Design review of the part built by this model. Coordinates are the model's own, in mm. A direction names the side the tool comes from. Coordinates: 2 decimals unless noted, no trailing zeros. Loops run counter-clockwise (first coordinate to the right, second up) from the corner with the lowest first, then second, coordinate; pieces in that order, holes last. Notation, with made-up numbers: (37, -32) -> (68, -32) arc R19 ccw to (68, -27) -> close; hole circle Ø2 at (2, 23). An arc over 180 degrees is marked (long way). Use a Markdown table: item, result. Add a question column.
Q1. Take a section at C-C on y = -12. Write out the cut boundary in (x, z) (3 decimals).
Q2. Take a section at D-D on z = 4.75. Write out the cut boundary in (x, y).
Q3. For probe 1 along Y at (x, z) = (19.5, -6); probe 2 along Z at (x, y) = (-4, -34); probe 3 along X at (y, z) = (-42, -5.25), list the stretches that pass through material, from the lowest coordinate up.
Q4. For faces 1 (the face through (11, -48, 9.525)), 2 (the face through (-9.516, -25.044, 0.419)), 3 (the face through (12, -50.8, 0)), list the 3-axis set-ups (+Z, -Z, +X, -X, +Y, -Y) from which the entire face can be reached by the end or side of a thin tool; tool diameter is ignored.
Q5. Take a section at B-B on x = 5. Write out the cut boundary in (y, z) (3 decimals), plus the area to 3 significant figures.
Q6. Clearance check with flat-ended pins moving along their axes: pin 1 Ø1.5 at (x, y) = (1.5, -31) entering from +Z; pin 2 Ø5 at (x, y) = (3, -41.5) entering from -Z; pin 3 Ø9.5 at (x, z) = (19.5, 4) entering from +Y. State where each tip first meets the part, or that it passes through.
Q7. Take a section at A-A on z = 0. Write out the cut boundary in (x, y) (3 decimals).
from build123d import *

# Parameters (mm, degrees)
F0_R     = 9.525
F1_DEPTH = 50.8
F3_DEPTH = 6.35
F4_W     = 3.175
F4_H     = 6.35
F5_DEPTH = 0.381


with BuildPart() as f1:
    # F0 (on Front) → F1 (new body)
    with BuildSketch(Plane.XZ):
        Circle(F0_R)
    extrude(amount=F1_DEPTH)

    # F2 (on face) → F3 (join)
    with BuildSketch(Plane.XZ.offset(50.8)):
        with BuildLine():
            Line((0, -9.525), (25.4, -9.525))
            ThreePointArc((25.4, -9.525), (34.925, 0), (25.4, 9.525))
            Line((25.4, 9.525), (0, 9.525))
            ThreePointArc((0, 9.525), (9.525, 0), (0, -9.525))
        make_face()
    extrude(amount=-F3_DEPTH)

    # F4 (on face) → F5 (join)
    with BuildSketch(Plane.XY.offset(9.525)):
        with Locations((23.8125, -47.625)):
            Rectangle(F4_W, F4_H)
    extrude(amount=F5_DEPTH)


solid = f1.part
Answer list:
| question | item | result |
|---|---|---|
| 1 | outline | circle Ø19.05 at (0, 0) |
| 2 | outline | (-8.26, -50.8) -> (33.66, -50.8) -> (33.66, -44.45) -> (8.26, -44.45) -> (8.26, 0) -> (-8.26, 0) -> close |
| 3 | probe 1 | -50.8 to -44.45 |
| 3 | probe 2 | -8.64 to 8.64 |
| 3 | probe 3 | -7.95 to 7.95 |
| 4 | face 1 | +Z, -X, +Y, -Y |
| 4 | face 2 | +Y |
| 4 | face 3 | +Z, -Z, +X, -X, -Y |
| 5 | outline | (-50.8, -9.525) -> (-44.45, -9.525) -> (-44.45, -8.107) -> (0, -8.107) -> (0, 8.107) -> (-44.45, 8.107) -> (-44.45, 9.525) -> (-50.8, 9.525) -> close |
| 5 | area | 842 mm² |
| 6 | pin 1 | z = 9.5 |
| 6 | pin 2 | z = -9.51 |
| 6 | pin 3 | y = -44.45 |
| 7 | outline | (-9.525, -50.8) -> (34.925, -50.8) -> (34.925, -44.45) -> (9.525, -44.45) -> (9.525, 0) -> (-9.525, 0) -> close |
